Could you check a few things on this model? Use its own coordinates, in mm. Face numbers are marked on the shaded views. A direction names the side the tool comes from. Coordinates: 2 decimals unless noted, no trailing zeros. Loops run counter-clockwise (first coordinate to the right, second up) from the corner with the lowest first, then second, coordinate; pieces in that order, holes last. Notation, with made-up numbers: (62.5, -23) -> (111.5, -23) arc R20 ccw to (111.5, -2) -> close; hole circle Ø8 at (63.5, 38.5). An arc over 180 degrees is marked (long way). One line per question, with ' | ' between items.
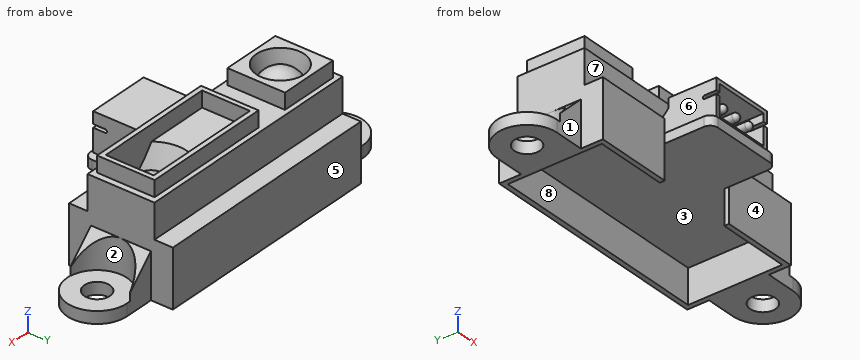
from build123d import *

# Parameters (mm, degrees)
SKETCH2_R                = 1.6
BOSS_EXTRUDE1_DEPTH      = 7.2
CUT_EXTRUDE1_DEPTH       = 84.563926387
SKETCH5_R                = 3.75
CUT_EXTRUDE2_DEPTH       = 87.349960246
SKETCH6_W                = 29.5
SKETCH6_H                = 8.4
BOSS_EXTRUDE2_DEPTH      = 4.3
SKETCH7_W                = 7.5
SKETCH7_H                = 7.2
SKETCH7_R                = 2.5
SKETCH7_W_2              = 16.3
SKETCH7_W_3              = 15.1
SKETCH7_H_2              = 6
BOSS_EXTRUDE3_DEPTH      = 2
CHAMFER1_SIZE2           = 2
CHAMFER1_SIZE            = 0.5
SKETCH8_R                = 2.5
CUT_EXTRUDE3_DEPTH       = 3
CHAMFER2_SIZE            = 2
CHAMFER2_SIZE_2          = 3.464101615
SKETCH9_W                = 28.3
SKETCH9_H                = 11.8
CUT_EXTRUDE4_DEPTH       = 5.5
BOSS_EXTRUDE4_DEPTH      = 1.2
FILLET1_R                = 1
BOSS_EXTRUDE5_DEPTH      = 3.95
BOSS_EXTRUDE5_DEPTH_BACK = 3.95
SKETCH17_W               = 6.9
SKETCH17_H               = 3.8
CUT_EXTRUDE5_DEPTH       = 5.8
SKETCH18_R               = 0.5
BOSS_EXTRUDE6_DEPTH      = 5.5
FILLET2_R                = 0.5


# Some blends are built 0.0001 mm under size
with BuildPart() as part:
    # Sketch2 → Boss-Extrude1 (new body)
    with BuildSketch(Plane.XY):
        with BuildLine():
            Line((-74.731926848, 25.724226739), (-45.231926848, 25.724226739))
            Line((-45.231926848, 25.724226739), (-45.231926848, 22.974226739))
            Line((-45.231926848, 22.974226739), (-41.481926848, 22.974226739))
            ThreePointArc((-41.481926848, 22.974226739), (-37.731926848, 19.224226739), (-41.481926848, 15.474226739))
            Line((-41.481926848, 15.474226739), (-45.231926848, 15.474226739))
            Line((-45.231926848, 15.474226739), (-45.231926848, 12.724226739))
            Line((-45.231926848, 12.724226739), (-54.931926848, 12.724226739))
            Line((-54.931926848, 12.724226739), (-54.931926848, 15.024226739))
            Line((-54.931926848, 15.024226739), (-65.031926848, 15.024226739))
            Line((-65.031926848, 15.024226739), (-65.031926848, 12.724226739))
            Line((-65.031926848, 12.724226739), (-74.731926848, 12.724226739))
            Line((-74.731926848, 12.724226739), (-74.731926848, 15.474226739))
            Line((-74.731926848, 15.474226739), (-78.481926848, 15.474226739))
            ThreePointArc((-78.481926848, 15.474226739), (-82.231926848, 19.224226739), (-78.481926848, 22.974226739))
            Line((-78.481926848, 22.974226739), (-74.731926848, 22.974226739))
            Line((-74.731926848, 22.974226739), (-74.731926848, 25.724226739))
        make_face()
        with Locations((-78.481926848, 19.224226739)):
            Circle(SKETCH2_R, mode=Mode.SUBTRACT)
        with Locations((-41.481926848, 19.224226739)):
            Circle(SKETCH2_R, mode=Mode.SUBTRACT)
    extrude(amount=BOSS_EXTRUDE1_DEPTH)

    # Sketch4 → Cut-Extrude1 (cut, through all)
    with BuildSketch(Plane.XZ.offset(-12.724226739)):
        Polygon((-74.731926848, 5.7), (-77.981926848, 2.5), (-77.981926848, 1.5), (-84.83036896, 1.5), (-84.83036896, 9.527639916), (-74.731926848, 9.527639916), align=None)
        Polygon((-45.231926848, 9.527639916), (-45.231926848, 5.7), (-41.981926848, 2.5), (-41.981926848, 1.5), (-35.133484736, 1.5), (-35.133484736, 9.527639916), align=None)
    extrude(amount=-CUT_EXTRUDE1_DEPTH, mode=Mode.SUBTRACT)

    # Sketch5 → Cut-Extrude2 (cut, through all)
    with BuildSketch(Plane.XY.offset(1.5)):
        with Locations((-78.481926848, 19.224226739)):
            Circle(SKETCH5_R)
        with Locations((-41.481926848, 19.224226739)):
            Circle(SKETCH5_R)
    extrude(amount=CUT_EXTRUDE2_DEPTH, mode=Mode.SUBTRACT)

    # Sketch6 → Boss-Extrude2 (add)
    with BuildSketch(Plane.XY.offset(7.2)):
        with Locations((-59.981926848, 19.224226739)):
            Rectangle(SKETCH6_W, SKETCH6_H)
    extrude(amount=BOSS_EXTRUDE2_DEPTH)

    # Sketch7 → Boss-Extrude3 (add)
    # profile 1 of 2: a face of its own
    with BuildSketch(Plane.XY.offset(11.5)):
        with Locations((-70.206926848, 19.224226739)):
            Rectangle(SKETCH7_W, SKETCH7_H)
        with Locations((-70.231926848, 19.224226739)):
            Circle(SKETCH7_R, mode=Mode.SUBTRACT)
    # profile 2 of 2: a face of its own
    with BuildSketch(Plane.XY.offset(11.5)):
        with Locations((-54.156926848, 19.224226739)):
            Rectangle(SKETCH7_W_2, SKETCH7_H)
        with Locations((-54.156926848, 19.224226739)):
            Rectangle(SKETCH7_W_3, SKETCH7_H_2, mode=Mode.SUBTRACT)
    extrude(amount=BOSS_EXTRUDE3_DEPTH)

    # Chamfer1
    chamfer1_edges = [part.edges().sort_by_distance(p)[0] for p in [
        (-72.731926848, 19.224226739, 13.5),
    ]]
    chamfer1_side = [part.faces().sort_by_distance(p)[0] for p in [
        (-72.741926848, 19.224226739, 13.5),
    ]]
    chamfer(chamfer1_edges, length=CHAMFER1_SIZE - 0.0001, length2=CHAMFER1_SIZE2 - 0.0001, reference=chamfer1_side[0])  # a hair under: the kernel refuses the full size

    # Sketch8 → Cut-Extrude3 (cut)
    with BuildSketch(Plane.XY.offset(11.5)):
        with Locations((-50.231926848, 18.99663901)):
            Circle(SKETCH8_R)
    extrude(amount=-CUT_EXTRUDE3_DEPTH, mode=Mode.SUBTRACT)

    # Chamfer2
    # the kernel refuses this chamfer: 3.464101615, 2 mm, written as the material it takes off along each edge
    with BuildSketch(Plane(origin=(-50.231926848, 18.99663901, 11.5), x_dir=(1, 0, 0), z_dir=(0, -1, 0))) as chamfer2_piece_1_section:
        Polygon((2.5 + CHAMFER2_SIZE, 0), (2.5, -CHAMFER2_SIZE_2), (2.5, 0), align=None)
    chamfer2_piece_1 = revolve(axis=Axis((-50.231926848, 18.99663901, 11.5), (0, 0, 1)), mode=Mode.PRIVATE)
    chamfer2_piece_1 = split(chamfer2_piece_1, bisect_by=Plane(origin=(-53.833665029, 16.224226739, 10.018611703), z_dir=(0, 1, 0)), keep=Keep.TOP, mode=Mode.PRIVATE)
    chamfer2_piece_1 = split(chamfer2_piece_1, bisect_by=Plane(origin=(-46.606926848, 18.99663901, 10.018611703), z_dir=(-1, 0, 0)), keep=Keep.TOP, mode=Mode.PRIVATE)
    chamfer2_piece_1 = split(chamfer2_piece_1, bisect_by=Plane(origin=(-53.833665029, 22.224226739, 10.018611703), z_dir=(0, -1, 0)), keep=Keep.TOP, mode=Mode.PRIVATE)
    chamfer2_piece_1 = split(chamfer2_piece_1, bisect_by=Plane(origin=(-53.833665029, 18.99663901, 8.5), z_dir=(0, 0, 1)), keep=Keep.TOP, mode=Mode.PRIVATE)
    add(chamfer2_piece_1, mode=Mode.SUBTRACT)

    # Sketch9 → Cut-Extrude4 (cut)
    with BuildSketch(Plane(origin=(0, 0, 0), x_dir=(-1, 0, 0), z_dir=(0, 0, -1))):
        with Locations((59.981926848, 19.224226739)):
            Rectangle(SKETCH9_W, SKETCH9_H)
    extrude(amount=-CUT_EXTRUDE4_DEPTH, mode=Mode.SUBTRACT)

    # Sketch10 → Boss-Extrude4 (add)
    with BuildSketch(Plane(origin=(0, 0, 5.5), x_dir=(-1, 0, 0), z_dir=(0, 0, -1))):
        Polygon((54.931926848, 13.324226739), (54.931926848, 6.824226739), (65.031926848, 6.824226739), (65.031926848, 13.324226739), (74.131926848, 13.324226739), (74.131926848, 25.124226739), (45.831926848, 25.124226739), (45.831926848, 13.324226739), align=None)
    extrude(amount=BOSS_EXTRUDE4_DEPTH)

    # Sketch11 → Revolve1 (revolve)
    with BuildSketch(Plane(origin=(0, 18.99663901, 0), x_dir=(1, 0, 0), z_dir=(0, 1, 0))):
        with BuildLine():
            Line((-50.231926848, -8.5), (-47.463977656, -8.5))
            ThreePointArc((-47.463977656, -8.5), (-48.524476795, -9.947681814), (-50.231926848, -10.5))
            Line((-50.231926848, -10.5), (-50.231926848, -8.5))
        make_face()
    revolve(axis=Axis((-50.231926848, 18.99663901, 8.5), (0, 0, 1)))

    # Sketch14 → Revolve2 (revolve)
    with BuildSketch(Plane(origin=(0, 19.224226739, 0), x_dir=(-1, 0, 0), z_dir=(0, -1, 0)), mode=Mode.PRIVATE) as revolve2_sk:
        with BuildLine():
            Line((70.231926848, -11.5), (72.731926848, -11.5))
            ThreePointArc((72.731926848, -11.5), (71.689664822, -12.596229956), (70.231926848, -13))
            Line((70.231926848, -13), (70.231926848, -11.5))
        make_face()
    revolve(revolve2_sk.sketch.rotate(Axis((-70.231926848, 19.224226739, 11.5), (0, 0, 1)), 180), axis=Axis((-70.231926848, 19.224226739, 11.5), (0, 0, 1)))

    # Fillet1
    fillet1_edges = [part.edges().sort_by_distance(p)[0] for p in [
        (-65.031926848, 6.824226739, 4.9),
        (-54.931926848, 6.824226739, 4.9),
    ]]
    fillet(fillet1_edges, radius=FILLET1_R)

    # Sketch16 → Boss-Extrude5 (add, two sides: drawn at the far end of the back side and taken through both)
    with BuildSketch(Plane(origin=(-59.981926848, 0, 0), x_dir=(0, 0, -1), z_dir=(1, 0, 0)).offset(-BOSS_EXTRUDE5_DEPTH_BACK)):
        with BuildLine():
            Line((-8.384982209, 8.613050121), (-8.384982209, 7.113050121))
            Line((-8.384982209, 7.113050121), (-5.5, 7.113050121))
            Line((-5.5, 7.113050121), (-5.5, 14.713050121))
            Line((-5.5, 14.713050121), (-7.5, 14.713050121))
            Line((-7.5, 14.713050121), (-9.1, 13.113050121))
            Line((-9.1, 13.113050121), (-10.3, 13.113050121))
            Line((-10.3, 13.113050121), (-10.3, 7.113050121))
            Line((-10.3, 7.113050121), (-8.815017791, 7.113050121))
            Line((-8.815017791, 7.113050121), (-8.815017791, 8.613050121))
            ThreePointArc((-8.815017791, 8.613050121), (-8.6, 8.828067912), (-8.384982209, 8.613050121))
        make_face()
    extrude(amount=BOSS_EXTRUDE5_DEPTH + BOSS_EXTRUDE5_DEPTH_BACK)

    # Sketch17 → Cut-Extrude5 (cut)
    with BuildSketch(Plane.XZ.offset(-7.113050121)):
        with Locations((-59.981926848, 7.9)):
            Rectangle(SKETCH17_W, SKETCH17_H)
    extrude(amount=-CUT_EXTRUDE5_DEPTH, mode=Mode.SUBTRACT)

    # Sketch18 → Boss-Extrude6 (add)
    with BuildSketch(Plane.XZ.offset(-12.913050121)):
        with Locations(Location((-59.981926848, 7.9, 0), (0, 0, 270))):
            Circle(SKETCH18_R)
        with Locations(Location((-57.981926848, 7.9, 0), (0, 0, 270))):
            Circle(SKETCH18_R)
        with Locations(Location((-61.981926848, 7.9, 0), (0, 0, 270))):
            Circle(SKETCH18_R)
    extrude(amount=BOSS_EXTRUDE6_DEPTH)

    # Fillet2
    fillet2_edges = [part.edges().sort_by_distance(p)[0] for p in [
        (-59.981926848, 7.413050121, 8.4),
        (-57.981926848, 7.413050121, 8.4),
        (-61.981926848, 7.413050121, 8.4),
    ]]
    fillet(fillet2_edges, radius=FILLET2_R)


solid = part.part
1) On a 3-axis mill with a long thin cutter (end or side, diameter ignored), from which of +Z, -Z, +X, -X, +Y, -Y can I reach the whole of each face in a straight line? I mean the marked faces 1, 2, 3 and 4. Say none if no direction works.
Data:
face 1: +Z, -Z, -X, -Y | face 2: +Z, +X | face 3: -Z | face 4: +Z, -Z, +X, -Y
2) We'd pull the mould along Y, two halves only. Please class the marked faces 5, 6, 7 and 8: pulls with the +Y half, pulls with the -Y half, needs draft (parallel to the pull), parting line crosses it, or undercut.
Data:
face 5: pulls with the +Y half | face 6: needs draft | face 7: undercut | face 8: undercut
3) I need wall thicknesses on line 1 along X through (y, z) = (14.5, 5.75); line 2 along Y through (x, z) = (-61.5, 10); line 3 along Y through (x, z) = (-53, 3.5). Which ranges of each line are inside material? Lowest first, please. Write a range as from..to.
Data:
line 1: -74.73..-65.03, -63.93..-56.03, -54.93..-45.23 | line 2: 7.11..13.11, 15.02..23.42 | line 3: 12.72..13.32, 25.12..25.72
4) If we section it at B-B on z = 12.25: Please give me the cut outline in (x, y), and give its area (3 significant figures).
Data:
outline: (-73.96, 15.62) -> (-66.46, 15.62) -> (-66.46, 22.82) -> (-73.96, 22.82) -> close; circle Ø3.84 at (-70.23, 19.22); (-62.31, 15.62) -> (-46.01, 15.62) -> (-46.01, 22.82) -> (-62.31, 22.82) -> close; hole circle Ø5.37 at (-70.23, 19.22); hole (-61.71, 16.22) -> (-46.61, 16.22) -> (-46.61, 22.22) -> (-61.71, 22.22) -> close | area: 69.7 mm²
5) I'm going to push flat-ended pins straight in: pin 1 Ø1.5 at (y, z) = (19, 9) entering from -X; pin 2 Ø6 at (y, z) = (22, 8.5) entering from +X; pin 3 Ø3 at (y, z) = (10, 8.5) entering from -X. Where does each tip first touch, or does it pass through?
Data:
pin 1: x = -74.73 | pin 2: x = -45.03 | pin 3: x = -63.93
6) If we section it at D-D on y = 24.25: Please give me the cut outline in (x, z), and give its area (3 significant figures).
Data:
outline: (-74.73, 0) -> (-74.13, 0) -> (-74.13, 4.3) -> (-45.83, 4.3) -> (-45.83, 0) -> (-45.23, 0) -> (-45.23, 7.2) -> (-74.73, 7.2) -> close | area: 90.7 mm²
7) If we section it at C-C on x = -41: Please give me the cut outline in (y, z).
Data:
outline: (15.51, 0) -> (17.7, 0) -> (17.7, 1.5) -> (15.51, 1.5) -> close; (20.75, 0) -> (22.94, 0) -> (22.94, 1.5) -> (20.75, 1.5) -> close
8) If we section it at A-A on y = 10.5: Please give me the cut outline in (x, z), and give its area (3 significant figures).
Data:
outline: (-65.03, 4.3) -> (-54.93, 4.3) -> (-54.93, 5.5) -> (-56.03, 5.5) -> (-56.03, 10.3) -> (-63.93, 10.3) -> (-63.93, 5.5) -> (-65.03, 5.5) -> close; circle Ø1 at (-61.98, 7.9); circle Ø1 at (-59.98, 7.9); circle Ø1 at (-57.98, 7.9); hole (-63.43, 6) -> (-56.53, 6) -> (-56.53, 9.8) -> (-63.43, 9.8) -> close | area: 26.2 mm²
